Source: CAD feature listing. Evaluate the final solid. Frame: model axes, mm. A direction names the side the tool comes from. Coordinates: 2 decimals unless noted, no trailing zeros. Loops run counter-clockwise (first coordinate to the right, second up) from the corner with the lowest first, then second, coordinate; pieces in that order, holes last.
Item 1: Pin query (flat end, axial travel): pin 1 Ø9.5 at (y, z) = (11, 12.7) entering from -X; pin 2 Ø4 at (x, y) = (14, 11) entering from +Z. Return the tip coordinate at first contact, or that it passes through.
Item 2: Reachability of faces 1 (the flat face through (19, 12, 23)), 2 (the flat face through (10, 22, 13)), 3 (the cylindrical face through (14.1, 14.5, 23)) from +Z, -Z, +X, -X, +Y, -Y: full face, straight path, thin tool, end or side. Return the list, or none.
Item 3: Section query C-C, the plane x = 5. Return the cut outline in (y, z).
Item 4: Section query A-A, the plane y = 11. Return the cut outline in (x, z), then the cut area to 3 significant figures.
Item 5: Line query: probe 1 along X at (y, z) = (11, 3.8); probe 2 along Y at (x, z) = (16.5, 12.7); probe 3 along Y at (x, z) = (5.75, 14.25). Output: solid intervals per line, ascending.
Item 6: Pull-direction query (X, two-part tool) for faces 4 (the cylindrical face through (15.717, 11.541, 1.521)), 5 (the flat face through (0, 11, 4)), 6 (the flat face through (21, 11, 4)); classes: +X half, -X half, draft (parallel to the pull), parting line (faces both ways), or undercut.
Item 7: Section query D-D, the plane z = 12.7. Return the cut outline in (x, y).
Item 8: Section query B-B, the plane z = 22.5. Return the cut outline in (x, y), then the cut area to 3 significant figures.
```python
from build123d import *

# Parameters (mm, degrees)
BOX_W           = 21
BOX_H           = 22
BOX_DEPTH       = 26
SKETCH_R        = 8
POCKET_DEPTH    = 21.001
SKETCH001_R     = 3.5
POCKET001_DEPTH = 23
SKETCH002_R     = 1.8
POCKET002_DEPTH = 5
SKETCH003_R     = 1.8
POCKET003_DEPTH = 22.001
SKETCH004_W     = 2
SKETCH004_H     = 11.298807
POCKET004_DEPTH = 21.001


with BuildPart() as part:
    # Box → Box (new body)
    with BuildSketch(Plane.XY):
        with Locations((10.5, 11)):
            Rectangle(BOX_W, BOX_H)
    extrude(amount=BOX_DEPTH)

    # Sketch → Pocket (cut, through all)
    with BuildSketch(Plane.YZ.offset(21)):
        with Locations((11, 12.7)):
            Circle(SKETCH_R)
    extrude(amount=-POCKET_DEPTH, mode=Mode.SUBTRACT)

    # Sketch001 → Pocket001 (cut)
    with BuildSketch(Plane.XY.offset(26)):
        with Locations((14, 11)):
            Circle(SKETCH001_R)
    extrude(amount=-POCKET001_DEPTH, mode=Mode.SUBTRACT)

    # Sketch002 → Pocket002 (cut)
    with BuildSketch(Plane.XY.offset(3)):
        with Locations((14, 11)):
            Circle(SKETCH002_R)
    extrude(amount=-POCKET002_DEPTH, mode=Mode.SUBTRACT)

    # Sketch003 → Pocket003 (cut, through all)
    with BuildSketch(Plane(origin=(0, 22, 0), x_dir=(-1, 0, 0), z_dir=(0, 1, 0))):
        with Locations((-5, 22.5)):
            Circle(SKETCH003_R)
    extrude(amount=-POCKET003_DEPTH, mode=Mode.SUBTRACT)

    # Sketch004 → Pocket004 (cut, through all)
    with BuildSketch(Plane.YZ.offset(21)):
        with Locations((11, 23.747477)):
            Rectangle(SKETCH004_W, SKETCH004_H)
    extrude(amount=-POCKET004_DEPTH, mode=Mode.SUBTRACT)


solid = part.part
```
Verdict:
1. pin 1: passes through
1. pin 2: stops at z = 3
2. face 1: +Z, +X, -X
2. face 2: +Z, -Z, +X, -X, +Y
2. face 3: +Z
3. outline: (0, 0) - (22, 0) - (22, 20.7) - (12, 20.7) - (12, 20.64) arc R8 cw (long way) to (10, 20.64) - (10, 20.7) - (0, 20.7) - close; (0, 24.3) - (10, 24.3) - (10, 26) - (0, 26) - close; (12, 24.3) - (22, 24.3) - (22, 26) - (12, 26) - close
4. outline: (0, 0) - (12.2, 0) - (12.2, 3) - (10.5, 3) - (10.5, 4.7) - (0, 4.7) - close; (15.8, 0) - (21, 0) - (21, 4.7) - (17.5, 4.7) - (17.5, 3) - (15.8, 3) - close
4. area: 76.0 mm2
5. probe 1: x = 0 to 10.5, 17.5 to 21
5. probe 2: y = 0 to 3, 19 to 22
5. probe 3: y = 0 to 3.15, 18.85 to 22
6. face 4: undercut
6. face 5: -X half
6. face 6: +X half
7. outline: (0, 0) - (21, 0) - (21, 3) - (0, 3) - close; (0, 19) - (21, 19) - (21, 22) - (0, 22) - close
8. outline: (0, 0) - (3.2, 0) - (3.2, 10) - (0, 10) - close; (0, 12) - (3.2, 12) - (3.2, 22) - (0, 22) - close; (6.8, 0) - (21, 0) - (21, 10) - (17.35, 10) arc R3.5 cw to (10.65, 10) - (6.8, 10) - close; (6.8, 12) - (10.65, 12) arc R3.5 cw to (17.35, 12) - (21, 12) - (21, 22) - (6.8, 22) - close
8. area: 323 mm2
